Source: CAD feature listing. Evaluate the final solid. Frame: model axes, mm. A direction names the side the tool comes from. Coordinates: 2 decimals unless noted, no trailing zeros. Loops run counter-clockwise (first coordinate to the right, second up) from the corner with the lowest first, then second, coordinate; pieces in that order, holes last. Notation, with made-up numbers: (28, -40) -> (48, -40) arc R23 cw to (48, -4) -> close; hole circle Ø11 at (42, -39.75). An arc over 180 degrees is marked (long way). Answer as CSV lines item,"result".
from build123d import *

# Parameters (mm, degrees)
F0_W     = 40
F0_H     = 5
F1_DEPTH = 25
F2_R     = 15
F3_R     = 25
F4_R     = 2.49999
F5_R     = 2
F6_SIZE  = 1


# Not quite as in the source:
# - a fillet or chamfer is up to 0.001 mm smaller than in the source, because OpenCascade refuses the exact size


with BuildPart() as f1:
    # F0 (on Top) → F1 (new body)
    with BuildSketch(Plane.XY):
        Polygon((0, 5), (0, 0), (0, -50), (-50, -50), (-50, -55), (5, -55), (5, -50.3902277714), (5, 0.3902277714), (5, 5), align=None)
        Polygon((20, -12.5), (5, 5), (5, 0.3902277714), (17, -13.6097722286), (17, -36.3902277714), (5, -50.3902277714), (5, -55), (20, -37.5), align=None)
        with Locations((-20, 2.5)):
            Rectangle(F0_W, F0_H)
    extrude(amount=F1_DEPTH)

    # F2
    f2_edges = [f1.edges().sort_by_distance(p)[0] for p in [
        (0, -50, 12.5),
    ]]
    fillet(f2_edges, radius=F2_R)

    # F3
    f3_edges = [f1.edges().sort_by_distance(p)[0] for p in [
        (5, -55, 12.5),
        (20, -37.5, 12.5),
        (20, -12.5, 12.5),
        (5, 5, 12.5),
        (17, -36.390228, 12.5),
        (17, -13.609772, 12.5),
    ]]
    fillet(f3_edges, radius=F3_R)

    # F4 (radius 2.5 in the source; OpenCascade refuses exactly that, so slightly less here)
    f4_edges = [f1.edges().sort_by_distance(p)[0] for p in [
        (-50, -55, 12.5),
        (-50, -50, 12.5),
        (-40, 0, 12.5),
        (-40, 5, 12.5),
    ]]
    fillet(f4_edges, radius=F4_R)

    # F5
    f5_edges = [f1.edges().sort_by_distance(p)[0] for p in [
        (5, -50.390228, 12.5),
        (5, 0.390228, 12.5),
    ]]
    fillet(f5_edges, radius=F5_R)

    # F6
    f6_edges = [f1.edges().sort_by_distance(p)[0] for p in [
        (9.749964, -5.151397, 25),
        (6.306108, -3.140517, 25),
        (15.447125, -14.184218, 25),
        (5, -25, 25),
        (17, -25, 25),
        (6.306108, -46.859483, 25),
        (15.447125, -35.815782, 25),
        (9.749964, -44.848603, 25),
        (-21.999192, 5, 25),
        (-39.26777, 4.26777, 25),
        (3.948047, 2.712822, 25),
        (-40, 2.5, 25),
        (13.232229, -4.604267, 25),
        (-39.26777, 0.73223, 25),
        (18.447125, -13.074446, 25),
        (-18.750005, 0, 25),
        (20, -25, 25),
        (0, -17.5, 25),
        (18.447125, -36.925554, 25),
        (-4.393398, -45.606602, 25),
        (13.232229, -45.395733, 25),
        (-31.250005, -50, 25),
        (3.948047, -52.712822, 25),
        (-49.26777, -50.73223, 25),
        (-26.999192, -55, 25),
        (-50, -52.5, 25),
        (-49.26777, -54.26777, 25),
        (9.749964, -5.151397, 0),
        (6.306108, -3.140517, 0),
        (15.447125, -14.184218, 0),
        (5, -25, 0),
        (17, -25, 0),
        (6.306108, -46.859483, 0),
        (15.447125, -35.815782, 0),
        (9.749964, -44.848603, 0),
        (-21.999192, 5, 0),
        (-39.26777, 4.26777, 0),
        (3.948047, 2.712822, 0),
        (-40, 2.5, 0),
        (13.232229, -4.604267, 0),
        (-39.26777, 0.73223, 0),
        (18.447125, -13.074446, 0),
        (-18.750005, 0, 0),
        (20, -25, 0),
        (0, -17.5, 0),
        (18.447125, -36.925554, 0),
        (-4.393398, -45.606602, 0),
        (13.232229, -45.395733, 0),
        (-31.250005, -50, 0),
        (3.948047, -52.712822, 0),
        (-49.26777, -50.73223, 0),
        (-26.999192, -55, 0),
        (-50, -52.5, 0),
        (-49.26777, -54.26777, 0),
    ]]
    chamfer(f6_edges, length=F6_SIZE)


solid = f1.part
(1) Cut plane C-C (x = -44.5). Return the cut outline in (y, z).
Computed values:
outline,"(-55, 1) -> (-54, 0) -> (-51, 0) -> (-50, 1) -> (-50, 24) -> (-51, 25) -> (-54, 25) -> (-55, 24) -> close"
(2) Pin query (flat end, axial travel): pin 1 Ø1.5 at (y, z) = (-31.5, 9) entering from -X; pin 2 Ø10 at (x, y) = (-20.5, -42) entering from +Z. Return the tip coordinate at first contact, or that it passes through.
Computed values:
pin 1,"x = 0"
pin 2,"through"
(3) Cut plane A-A (x = -35). Return the cut outline in (y, z).
Computed values:
outline,"(-55, 1) -> (-54, 0) -> (-51, 0) -> (-50, 1) -> (-50, 24) -> (-51, 25) -> (-54, 25) -> (-55, 24) -> close; (0, 1) -> (1, 0) -> (4, 0) -> (5, 1) -> (5, 24) -> (4, 25) -> (1, 25) -> (0, 24) -> close"
(4) Draft query along X for faces 1 (the conical face through (6.285, -47.022, 0.84)), 2 (the flat face through (12.85, -45.09, 0.51)), 3 (the flat face through (2, -29, 25)). Return one class per face: released by +X, released by -X, zero draft, split by the parting line, or undercut.
Computed values:
face 1,"undercut"
face 2,"released by +X"
face 3,"zero draft"
(5) Access query for faces 4 (the flat face through (9.73, -5.13, 12.34)), 5 (the conical face through (-4.16, -45.6, 0.84)), 6 (the flat face through (10.152, -45.158, 24.507)), 7 (the flat face through (10.107, -4.81, 0.507)), 8 (the cylindrical face through (18.404, -37.042, 12.661)). Directions: +Z, -Z, +X, -X, +Y, -Y. A direction counts if a zero-diameter tool reaches every point of the face in a straight line with its end or side. Return the directions, or none.
Computed values:
face 4,"+Z, -Z"
face 5,"-Z, -X"
face 6,"+Z"
face 7,"-Z"
face 8,"+Z, -Z, +X, -Y"
(6) Material intervals for L1, parallel to Y at x = -25, z = 16.5; L2, parallel to X at y = -34, z = 17.5; L3, parallel to X at y = -13, z = 12.75, sorted ascending. Write a range as [from, to].
Computed values:
L1,"[-55, -50], [0, 5]"
L2,"[0, 5], [16.04, 19.33]"
L3,"[0, 5], [14.97, 18.42]"
